Input: part model. Units: mm. Frame: model coordinates. A direction names the side the tool comes from. Coordinates: 2 decimals unless noted, no trailing zeros. Order: outer loops, then holes, each group sorted by start corner. A loop starts at its lowest first (then second) coordinate and runs counter-clockwise, first axis right, second up.
from build123d import *

# Parameters (mm, degrees)
SKETCH1_W                  = 80
SKETCH1_H                  = 270
BOSS_EXTRUDE1_DEPTH        = 5
SKETCH2_W                  = 65
SKETCH2_H                  = 45
BOSS_EXTRUDE3_DEPTH        = 2
LPATTERN1_COUNT            = 5
LPATTERN1_PITCH            = 50
SKETCH3_W                  = 70
SKETCH3_H                  = 48.748964222
BOSS_EXTRUDE8_DEPTH        = 25
LPATTERN5_COUNT            = 5
LPATTERN5_PITCH            = 50
LPATTERN6_COUNT            = 3
LPATTERN6_PITCH            = 80
LPATTERN6_COPY_1_SKETCH_W  = 65
LPATTERN6_COPY_1_SKETCH_H  = 45
LPATTERN6_COPY_1_DEPTH     = 2
LPATTERN6_COPY_2_SKETCH_W  = 65
LPATTERN6_COPY_2_SKETCH_H  = 45
LPATTERN6_COPY_2_DEPTH     = 2
LPATTERN6_COPY_3_SKETCH_W  = 65
LPATTERN6_COPY_3_SKETCH_H  = 45
LPATTERN6_COPY_3_DEPTH     = 2
LPATTERN6_COPY_4_SKETCH_W  = 65
LPATTERN6_COPY_4_SKETCH_H  = 45
LPATTERN6_COPY_4_DEPTH     = 2
LPATTERN6_COPY_5_SKETCH_W  = 65
LPATTERN6_COPY_5_SKETCH_H  = 45
LPATTERN6_COPY_5_DEPTH     = 2
LPATTERN6_COPY_6_SKETCH_W  = 65
LPATTERN6_COPY_6_SKETCH_H  = 45
LPATTERN6_COPY_6_DEPTH     = 2
LPATTERN6_COPY_7_SKETCH_W  = 65
LPATTERN6_COPY_7_SKETCH_H  = 45
LPATTERN6_COPY_7_DEPTH     = 2
LPATTERN6_COPY_8_SKETCH_W  = 65
LPATTERN6_COPY_8_SKETCH_H  = 45
LPATTERN6_COPY_8_DEPTH     = 2
LPATTERN6_COPY_9_SKETCH_W  = 70
LPATTERN6_COPY_9_SKETCH_H  = 48.748964222
LPATTERN6_COPY_9_DEPTH     = 25
LPATTERN6_COPY_10_SKETCH_W = 70
LPATTERN6_COPY_10_SKETCH_H = 48.748964222
LPATTERN6_COPY_10_DEPTH    = 25
LPATTERN6_COPY_11_SKETCH_W = 70
LPATTERN6_COPY_11_SKETCH_H = 48.748964222
LPATTERN6_COPY_11_DEPTH    = 25
LPATTERN6_COPY_12_SKETCH_W = 70
LPATTERN6_COPY_12_SKETCH_H = 48.748964222
LPATTERN6_COPY_12_DEPTH    = 25
LPATTERN6_COPY_13_SKETCH_W = 70
LPATTERN6_COPY_13_SKETCH_H = 48.748964222
LPATTERN6_COPY_13_DEPTH    = 25
LPATTERN6_COPY_14_SKETCH_W = 70
LPATTERN6_COPY_14_SKETCH_H = 48.748964222
LPATTERN6_COPY_14_DEPTH    = 25
LPATTERN6_COPY_15_SKETCH_W = 70
LPATTERN6_COPY_15_SKETCH_H = 48.748964222
LPATTERN6_COPY_15_DEPTH    = 25
LPATTERN6_COPY_16_SKETCH_W = 70
LPATTERN6_COPY_16_SKETCH_H = 48.748964222
LPATTERN6_COPY_16_DEPTH    = 25


with BuildPart() as part:
    # Sketch1 → Boss-Extrude1 (new body)
    with BuildSketch(Plane(origin=(0, 0, 0), x_dir=(1, 0, 0), z_dir=(0, 1, 0))):
        Rectangle(SKETCH1_W, SKETCH1_H)
    boss_extrude1 = extrude(amount=BOSS_EXTRUDE1_DEPTH)

    # Sketch2 → Boss-Extrude3 (add)
    with BuildSketch(Plane(origin=(0, 5, 0), x_dir=(1, 0, 0), z_dir=(0, 1, 0))):
        with Locations((0, -100)):
            Rectangle(SKETCH2_W, SKETCH2_H)
    boss_extrude3 = extrude(amount=BOSS_EXTRUDE3_DEPTH)

    # LPattern1: Boss-Extrude3 ×5
    with Locations(*[(0, 0, -i * LPATTERN1_PITCH) for i in range(1, LPATTERN1_COUNT)]):
        add(boss_extrude3)

    # Sketch3 → Boss-Extrude8 (add)
    with BuildSketch(Plane(origin=(0, 7, 0), x_dir=(1, 0, 0), z_dir=(0, 1, 0))):
        with Locations((0, -99.635002086)):
            Rectangle(SKETCH3_W, SKETCH3_H)
    boss_extrude8 = extrude(amount=BOSS_EXTRUDE8_DEPTH)

    # LPattern5: Boss-Extrude8 ×5
    with Locations(*[(0, 0, -i * LPATTERN5_PITCH) for i in range(1, LPATTERN5_COUNT)]):
        add(boss_extrude8)

    # LPattern6: Boss-Extrude1, Boss-Extrude3, Boss-Extrude8 ×3
    with Locations(*[(-i * LPATTERN6_PITCH, 0, 0) for i in range(1, LPATTERN6_COUNT)]):
        add(boss_extrude1)
        add(boss_extrude3)
        add(boss_extrude8)

    # LPattern6 copy 1 sketch → LPattern6 copy 1 (add)
    with BuildSketch(Plane(origin=(-80, 5, -50), x_dir=(1, 0, 0), z_dir=(0, 1, 0))):
        with Locations((0, -100)):
            Rectangle(LPATTERN6_COPY_1_SKETCH_W, LPATTERN6_COPY_1_SKETCH_H)
    extrude(amount=LPATTERN6_COPY_1_DEPTH)

    # LPattern6 copy 2 sketch → LPattern6 copy 2 (add)
    with BuildSketch(Plane(origin=(-160, 5, -50), x_dir=(1, 0, 0), z_dir=(0, 1, 0))):
        with Locations((0, -100)):
            Rectangle(LPATTERN6_COPY_2_SKETCH_W, LPATTERN6_COPY_2_SKETCH_H)
    extrude(amount=LPATTERN6_COPY_2_DEPTH)

    # LPattern6 copy 3 sketch → LPattern6 copy 3 (add)
    with BuildSketch(Plane(origin=(-80, 5, -100), x_dir=(1, 0, 0), z_dir=(0, 1, 0))):
        with Locations((0, -100)):
            Rectangle(LPATTERN6_COPY_3_SKETCH_W, LPATTERN6_COPY_3_SKETCH_H)
    extrude(amount=LPATTERN6_COPY_3_DEPTH)

    # LPattern6 copy 4 sketch → LPattern6 copy 4 (add)
    with BuildSketch(Plane(origin=(-160, 5, -100), x_dir=(1, 0, 0), z_dir=(0, 1, 0))):
        with Locations((0, -100)):
            Rectangle(LPATTERN6_COPY_4_SKETCH_W, LPATTERN6_COPY_4_SKETCH_H)
    extrude(amount=LPATTERN6_COPY_4_DEPTH)

    # LPattern6 copy 5 sketch → LPattern6 copy 5 (add)
    with BuildSketch(Plane(origin=(-80, 5, -150), x_dir=(1, 0, 0), z_dir=(0, 1, 0))):
        with Locations((0, -100)):
            Rectangle(LPATTERN6_COPY_5_SKETCH_W, LPATTERN6_COPY_5_SKETCH_H)
    extrude(amount=LPATTERN6_COPY_5_DEPTH)

    # LPattern6 copy 6 sketch → LPattern6 copy 6 (add)
    with BuildSketch(Plane(origin=(-160, 5, -150), x_dir=(1, 0, 0), z_dir=(0, 1, 0))):
        with Locations((0, -100)):
            Rectangle(LPATTERN6_COPY_6_SKETCH_W, LPATTERN6_COPY_6_SKETCH_H)
    extrude(amount=LPATTERN6_COPY_6_DEPTH)

    # LPattern6 copy 7 sketch → LPattern6 copy 7 (add)
    with BuildSketch(Plane(origin=(-80, 5, -200), x_dir=(1, 0, 0), z_dir=(0, 1, 0))):
        with Locations((0, -100)):
            Rectangle(LPATTERN6_COPY_7_SKETCH_W, LPATTERN6_COPY_7_SKETCH_H)
    extrude(amount=LPATTERN6_COPY_7_DEPTH)

    # LPattern6 copy 8 sketch → LPattern6 copy 8 (add)
    with BuildSketch(Plane(origin=(-160, 5, -200), x_dir=(1, 0, 0), z_dir=(0, 1, 0))):
        with Locations((0, -100)):
            Rectangle(LPATTERN6_COPY_8_SKETCH_W, LPATTERN6_COPY_8_SKETCH_H)
    extrude(amount=LPATTERN6_COPY_8_DEPTH)

    # LPattern6 copy 9 sketch → LPattern6 copy 9 (add)
    with BuildSketch(Plane(origin=(-80, 7, -50), x_dir=(1, 0, 0), z_dir=(0, 1, 0))):
        with Locations((0, -99.635002086)):
            Rectangle(LPATTERN6_COPY_9_SKETCH_W, LPATTERN6_COPY_9_SKETCH_H)
    extrude(amount=LPATTERN6_COPY_9_DEPTH)

    # LPattern6 copy 10 sketch → LPattern6 copy 10 (add)
    with BuildSketch(Plane(origin=(-160, 7, -50), x_dir=(1, 0, 0), z_dir=(0, 1, 0))):
        with Locations((0, -99.635002086)):
            Rectangle(LPATTERN6_COPY_10_SKETCH_W, LPATTERN6_COPY_10_SKETCH_H)
    extrude(amount=LPATTERN6_COPY_10_DEPTH)

    # LPattern6 copy 11 sketch → LPattern6 copy 11 (add)
    with BuildSketch(Plane(origin=(-80, 7, -100), x_dir=(1, 0, 0), z_dir=(0, 1, 0))):
        with Locations((0, -99.635002086)):
            Rectangle(LPATTERN6_COPY_11_SKETCH_W, LPATTERN6_COPY_11_SKETCH_H)
    extrude(amount=LPATTERN6_COPY_11_DEPTH)

    # LPattern6 copy 12 sketch → LPattern6 copy 12 (add)
    with BuildSketch(Plane(origin=(-160, 7, -100), x_dir=(1, 0, 0), z_dir=(0, 1, 0))):
        with Locations((0, -99.635002086)):
            Rectangle(LPATTERN6_COPY_12_SKETCH_W, LPATTERN6_COPY_12_SKETCH_H)
    extrude(amount=LPATTERN6_COPY_12_DEPTH)

    # LPattern6 copy 13 sketch → LPattern6 copy 13 (add)
    with BuildSketch(Plane(origin=(-80, 7, -150), x_dir=(1, 0, 0), z_dir=(0, 1, 0))):
        with Locations((0, -99.635002086)):
            Rectangle(LPATTERN6_COPY_13_SKETCH_W, LPATTERN6_COPY_13_SKETCH_H)
    extrude(amount=LPATTERN6_COPY_13_DEPTH)

    # LPattern6 copy 14 sketch → LPattern6 copy 14 (add)
    with BuildSketch(Plane(origin=(-160, 7, -150), x_dir=(1, 0, 0), z_dir=(0, 1, 0))):
        with Locations((0, -99.635002086)):
            Rectangle(LPATTERN6_COPY_14_SKETCH_W, LPATTERN6_COPY_14_SKETCH_H)
    extrude(amount=LPATTERN6_COPY_14_DEPTH)

    # LPattern6 copy 15 sketch → LPattern6 copy 15 (add)
    with BuildSketch(Plane(origin=(-80, 7, -200), x_dir=(1, 0, 0), z_dir=(0, 1, 0))):
        with Locations((0, -99.635002086)):
            Rectangle(LPATTERN6_COPY_15_SKETCH_W, LPATTERN6_COPY_15_SKETCH_H)
    extrude(amount=LPATTERN6_COPY_15_DEPTH)

    # LPattern6 copy 16 sketch → LPattern6 copy 16 (add)
    with BuildSketch(Plane(origin=(-160, 7, -200), x_dir=(1, 0, 0), z_dir=(0, 1, 0))):
        with Locations((0, -99.635002086)):
            Rectangle(LPATTERN6_COPY_16_SKETCH_W, LPATTERN6_COPY_16_SKETCH_H)
    extrude(amount=LPATTERN6_COPY_16_DEPTH)


solid = part.part
Item 1: Pin query (flat end, axial travel): pin 1 Ø12.5 at (y, z) = (23.5, -52.5) entering from -X; pin 2 Ø2 at (x, y) = (-76.5, 19) entering from -Z; pin 3 Ø4 at (y, z) = (26.5, 31) entering from +X; pin 4 Ø12 at (x, y) = (-122, 6.5) entering from +Z. Return the tip coordinate at first contact, or that it passes through.
Response values:
pin 1: stops at x = -195
pin 2: stops at z = -124.74
pin 3: stops at x = 35
pin 4: stops at z = 135
Item 2: Cut plane A-A on z = -31.5. Return loops of the section in (x, y).
Response values:
outline: (-200, 0) - (40, 0) - (40, 5) - (32.5, 5) - (32.5, 7) - (35, 7) - (35, 32) - (-35, 32) - (-35, 7) - (-32.5, 7) - (-32.5, 5) - (-47.5, 5) - (-47.5, 7) - (-45, 7) - (-45, 32) - (-115, 32) - (-115, 7) - (-112.5, 7) - (-112.5, 5) - (-127.5, 5) - (-127.5, 7) - (-125, 7) - (-125, 32) - (-195, 32) - (-195, 7) - (-192.5, 7) - (-192.5, 5) - (-200, 5) - close
Item 3: Ray query, probe 1 along Z at (x, y) = (16, 28); probe 2 along X at (y, z) = (16, 55). Return the intervals inside material, ascending.
Response values:
probe 1: z = -124.74 to -75.99, -74.74 to -25.99, -24.74 to 24.01, 25.26 to 74.01, 75.26 to 124.01
probe 2: x = -195 to -125, -115 to -45, -35 to 35
Item 4: Access query for faces 1 (the face through (35, 19, 100)), 2 (the face through (-83, 7, 123)), 3 (the face through (-160, 19, 25.261)), 4 (the face through (-45, 19, -100)). Directions: +Z, -Z, +X, -X, +Y, -Y. A direction counts if a zero-diameter tool reaches every point of the face in a straight line with its end or side. Return the directions, or none.
Response values:
face 1: +Z, -Z, +X, +Y
face 2: none
face 3: +X, -X, +Y
face 4: +Z, -Z, +Y
Item 5: Cut plane B-B on y = 14. Count the separate pieces of the cut face and the enclosed holes in it, then the cut area to 3 significant figures.
Response values:
separate pieces: 15
enclosed holes: 0
area: 51,200 mm2
Item 6: Draft query along Z for faces 5 (the face through (35, 19, -100)), 6 (the face through (-80, 19, 74.009)). Return one class per face: pulls with the +Z half, pulls with the -Z half, needs draft (parallel to the pull), parting line crosses it, or undercut.
Response values:
face 5: needs draft
face 6: undercut
